Work out the finished part from the listing and answer in its coordinate system (mm). A direction names the side the tool comes from. Round coordinates to 2 decimals unless told otherwise and drop trailing zeros. Order: outer loops, then holes, each group sorted by start corner. A loop starts at its lowest first (then second) coordinate and runs counter-clockwise, first axis right, second up. Notation, with made-up numbers: M 80,-20 L 108,-20 A31 ccw 108,14 Z; hole C 89,86.25 d6. An arc over 180 degrees is marked long. Return JSON: item names as keys, results as strings.
from build123d import *

# Parameters (mm, degrees)
CYLINDER074_R          = 2
CYLINDER074_DEPTH      = 10
CYLINDER073_R          = 2
CYLINDER073_DEPTH      = 10
CYLINDER075_R          = 2
CYLINDER075_DEPTH      = 10
CYLINDER076_R          = 2
CYLINDER076_DEPTH      = 10
BOX103_W               = 1
BOX103_H               = 100
BOX103_DEPTH           = 5
BOX102_W               = 1
BOX102_H               = 100
BOX102_DEPTH           = 5
BOX100_W               = 2
BOX100_H               = 2
BOX100_DEPTH           = 80
BOX100_PLACEMENT_ANGLE = 45
BOX101_W               = 2
BOX101_H               = 2
BOX101_DEPTH           = 80
BOX101_PLACEMENT_ANGLE = 45
BOX097_W               = 2
BOX097_H               = 2
BOX097_DEPTH           = 80
BOX097_PLACEMENT_ANGLE = 45
BOX096_W               = 2
BOX096_H               = 2
BOX096_DEPTH           = 80
BOX096_PLACEMENT_ANGLE = 45
BOX095_W               = 2
BOX095_H               = 2
BOX095_DEPTH           = 80
BOX095_PLACEMENT_ANGLE = 45
BOX094_W               = 2
BOX094_H               = 2
BOX094_DEPTH           = 80
BOX094_PLACEMENT_ANGLE = 45
BOX093_W               = 2
BOX093_H               = 2
BOX093_DEPTH           = 80
BOX093_PLACEMENT_ANGLE = 45
BOX092_W               = 2
BOX092_H               = 2
BOX092_DEPTH           = 80
BOX092_PLACEMENT_ANGLE = 45
BOX091_W               = 2
BOX091_H               = 2
BOX091_DEPTH           = 80
BOX091_PLACEMENT_ANGLE = 45
BOX090_W               = 2
BOX090_H               = 2
BOX090_DEPTH           = 80
BOX090_PLACEMENT_ANGLE = 45
BOX089_W               = 2
BOX089_H               = 2
BOX089_DEPTH           = 80
BOX089_PLACEMENT_ANGLE = 45
BOX088_W               = 2
BOX088_H               = 2
BOX088_DEPTH           = 80
BOX088_PLACEMENT_ANGLE = 45
BOX087_W               = 2
BOX087_H               = 2
BOX087_DEPTH           = 80
BOX087_PLACEMENT_ANGLE = 45
BOX086_W               = 2
BOX086_H               = 2
BOX086_DEPTH           = 80
BOX086_PLACEMENT_ANGLE = 45
BOX084_W               = 2
BOX084_H               = 2
BOX084_DEPTH           = 80
BOX084_PLACEMENT_ANGLE = 45
BOX085_W               = 2
BOX085_H               = 2
BOX085_DEPTH           = 80
BOX085_PLACEMENT_ANGLE = 45
BOX099_W               = 2
BOX099_H               = 2
BOX099_DEPTH           = 80
BOX099_PLACEMENT_ANGLE = 45
BOX098_W               = 2
BOX098_H               = 50
BOX098_DEPTH           = 50
PAD014_DEPTH           = 5
BOX083_W               = 2
BOX083_H               = 93
BOX083_DEPTH           = 130
CUT076_PLACEMENT_ANGLE = 90


with BuildPart() as cylinder043:
    # Cylinder074 → Cylinder074 (new body)
    with BuildSketch(Plane(origin=(102, 0, 27), x_dir=(1, 0, 0), z_dir=(0, -1, 0))):
        Circle(CYLINDER074_R)
    extrude(amount=CYLINDER074_DEPTH)


with BuildPart() as cylinder042:
    # Cylinder073 → Cylinder073 (new body)
    with BuildSketch(Plane(origin=(19.8, 0, 27), x_dir=(1, 0, 0), z_dir=(0, -1, 0))):
        Circle(CYLINDER073_R)
    extrude(amount=CYLINDER073_DEPTH)


with BuildPart() as cylinder044:
    # Cylinder075 → Cylinder075 (new body)
    with BuildSketch(Plane(origin=(102, 0, 143), x_dir=(1, 0, 0), z_dir=(0, -1, 0))):
        Circle(CYLINDER075_R)
    extrude(amount=CYLINDER075_DEPTH)


with BuildPart() as obj1:
    # Cylinder076 → Cylinder076 (new body)
    with BuildSketch(Plane(origin=(32.2, 0, 143), x_dir=(1, 0, 0), z_dir=(0, -1, 0))):
        Circle(CYLINDER076_R)
    extrude(amount=CYLINDER076_DEPTH)

    # Fusion045: union Cylinder043, Cylinder042, Cylinder044
    add(cylinder043.part)
    add(cylinder042.part)
    add(cylinder044.part)


with BuildPart() as obj1_1:
    # Fusion045 placement: moved
    add(obj1.part.moved(Location((0, 5, 0))))


with BuildPart() as cube094:
    # Box103 → Box103 (new body)
    with BuildSketch(Plane.XY.offset(125)):
        with Locations((0.5, 50)):
            Rectangle(BOX103_W, BOX103_H)
    extrude(amount=BOX103_DEPTH)


with BuildPart() as obj2:
    # Box102 → Box102 (new body)
    with BuildSketch(Plane.XY):
        with Locations((0.5, 50)):
            Rectangle(BOX102_W, BOX102_H)
    extrude(amount=BOX102_DEPTH)

    # Fusion044: union Cube094
    add(cube094.part)


with BuildPart() as cube091:
    # Box100 → Box100 (new body)
    with BuildSketch(Plane.XY):
        with Locations((1, 1)):
            Rectangle(BOX100_W, BOX100_H)
    extrude(amount=BOX100_DEPTH)


with BuildPart() as cube091_1:
    # Box100 placement: moved
    add(cube091.part.moved(Location((0, 90, 0))).rotate(Axis((0, 90, 0), (-1, 0, 0)), BOX100_PLACEMENT_ANGLE))


with BuildPart() as cube092:
    # Box101 → Box101 (new body)
    with BuildSketch(Plane.XY):
        with Locations((1, 1)):
            Rectangle(BOX101_W, BOX101_H)
    extrude(amount=BOX101_DEPTH)


with BuildPart() as cube092_1:
    # Box101 placement: moved
    add(cube092.part.moved(Location((0, 96, 0))).rotate(Axis((0, 96, 0), (-1, 0, 0)), BOX101_PLACEMENT_ANGLE))


with BuildPart() as cube088:
    # Box097 → Box097 (new body)
    with BuildSketch(Plane.XY):
        with Locations((1, 1)):
            Rectangle(BOX097_W, BOX097_H)
    extrude(amount=BOX097_DEPTH)


with BuildPart() as cube088_1:
    # Box097 placement: moved
    add(cube088.part.moved(Location((0, 78, 0))).rotate(Axis((0, 78, 0), (-1, 0, 0)), BOX097_PLACEMENT_ANGLE))


with BuildPart() as cube087:
    # Box096 → Box096 (new body)
    with BuildSketch(Plane.XY):
        with Locations((1, 1)):
            Rectangle(BOX096_W, BOX096_H)
    extrude(amount=BOX096_DEPTH)


with BuildPart() as cube087_1:
    # Box096 placement: moved
    add(cube087.part.moved(Location((0, 72, 0))).rotate(Axis((0, 72, 0), (-1, 0, 0)), BOX096_PLACEMENT_ANGLE))


with BuildPart() as cube086:
    # Box095 → Box095 (new body)
    with BuildSketch(Plane.XY):
        with Locations((1, 1)):
            Rectangle(BOX095_W, BOX095_H)
    extrude(amount=BOX095_DEPTH)


with BuildPart() as cube086_1:
    # Box095 placement: moved
    add(cube086.part.moved(Location((0, 66, 0))).rotate(Axis((0, 66, 0), (-1, 0, 0)), BOX095_PLACEMENT_ANGLE))


with BuildPart() as cube085:
    # Box094 → Box094 (new body)
    with BuildSketch(Plane.XY):
        with Locations((1, 1)):
            Rectangle(BOX094_W, BOX094_H)
    extrude(amount=BOX094_DEPTH)


with BuildPart() as cube085_1:
    # Box094 placement: moved
    add(cube085.part.moved(Location((0, 60, 0))).rotate(Axis((0, 60, 0), (-1, 0, 0)), BOX094_PLACEMENT_ANGLE))


with BuildPart() as cube084:
    # Box093 → Box093 (new body)
    with BuildSketch(Plane.XY):
        with Locations((1, 1)):
            Rectangle(BOX093_W, BOX093_H)
    extrude(amount=BOX093_DEPTH)


with BuildPart() as cube084_1:
    # Box093 placement: moved
    add(cube084.part.moved(Location((0, 54, 0))).rotate(Axis((0, 54, 0), (-1, 0, 0)), BOX093_PLACEMENT_ANGLE))


with BuildPart() as cube083:
    # Box092 → Box092 (new body)
    with BuildSketch(Plane.XY):
        with Locations((1, 1)):
            Rectangle(BOX092_W, BOX092_H)
    extrude(amount=BOX092_DEPTH)


with BuildPart() as cube083_1:
    # Box092 placement: moved
    add(cube083.part.moved(Location((0, 48, 0))).rotate(Axis((0, 48, 0), (-1, 0, 0)), BOX092_PLACEMENT_ANGLE))


with BuildPart() as cube082:
    # Box091 → Box091 (new body)
    with BuildSketch(Plane.XY):
        with Locations((1, 1)):
            Rectangle(BOX091_W, BOX091_H)
    extrude(amount=BOX091_DEPTH)


with BuildPart() as cube082_1:
    # Box091 placement: moved
    add(cube082.part.moved(Location((0, 42, 0))).rotate(Axis((0, 42, 0), (-1, 0, 0)), BOX091_PLACEMENT_ANGLE))


with BuildPart() as cube081:
    # Box090 → Box090 (new body)
    with BuildSketch(Plane.XY):
        with Locations((1, 1)):
            Rectangle(BOX090_W, BOX090_H)
    extrude(amount=BOX090_DEPTH)


with BuildPart() as cube081_1:
    # Box090 placement: moved
    add(cube081.part.moved(Location((0, 36, 0))).rotate(Axis((0, 36, 0), (-1, 0, 0)), BOX090_PLACEMENT_ANGLE))


with BuildPart() as cube080:
    # Box089 → Box089 (new body)
    with BuildSketch(Plane.XY):
        with Locations((1, 1)):
            Rectangle(BOX089_W, BOX089_H)
    extrude(amount=BOX089_DEPTH)


with BuildPart() as cube080_1:
    # Box089 placement: moved
    add(cube080.part.moved(Location((0, 30, 0))).rotate(Axis((0, 30, 0), (-1, 0, 0)), BOX089_PLACEMENT_ANGLE))


with BuildPart() as cube079:
    # Box088 → Box088 (new body)
    with BuildSketch(Plane.XY):
        with Locations((1, 1)):
            Rectangle(BOX088_W, BOX088_H)
    extrude(amount=BOX088_DEPTH)


with BuildPart() as cube079_1:
    # Box088 placement: moved
    add(cube079.part.moved(Location((0, 24, 0))).rotate(Axis((0, 24, 0), (-1, 0, 0)), BOX088_PLACEMENT_ANGLE))


with BuildPart() as cube078:
    # Box087 → Box087 (new body)
    with BuildSketch(Plane.XY):
        with Locations((1, 1)):
            Rectangle(BOX087_W, BOX087_H)
    extrude(amount=BOX087_DEPTH)


with BuildPart() as cube078_1:
    # Box087 placement: moved
    add(cube078.part.moved(Location((0, 18, 0))).rotate(Axis((0, 18, 0), (-1, 0, 0)), BOX087_PLACEMENT_ANGLE))


with BuildPart() as cube077:
    # Box086 → Box086 (new body)
    with BuildSketch(Plane.XY):
        with Locations((1, 1)):
            Rectangle(BOX086_W, BOX086_H)
    extrude(amount=BOX086_DEPTH)


with BuildPart() as cube077_1:
    # Box086 placement: moved
    add(cube077.part.moved(Location((0, 12, 0))).rotate(Axis((0, 12, 0), (-1, 0, 0)), BOX086_PLACEMENT_ANGLE))


with BuildPart() as cube075:
    # Box084 → Box084 (new body)
    with BuildSketch(Plane.XY):
        with Locations((1, 1)):
            Rectangle(BOX084_W, BOX084_H)
    extrude(amount=BOX084_DEPTH)


with BuildPart() as cube075_1:
    # Box084 placement: moved
    add(cube075.part.rotate(Axis((0, 0, 0), (-1, 0, 0)), BOX084_PLACEMENT_ANGLE))


with BuildPart() as cube076:
    # Box085 → Box085 (new body)
    with BuildSketch(Plane.XY):
        with Locations((1, 1)):
            Rectangle(BOX085_W, BOX085_H)
    extrude(amount=BOX085_DEPTH)


with BuildPart() as cube076_1:
    # Box085 placement: moved
    add(cube076.part.moved(Location((0, 6, 0))).rotate(Axis((0, 6, 0), (-1, 0, 0)), BOX085_PLACEMENT_ANGLE))


with BuildPart() as fusion043:
    # Box099 → Box099 (new body)
    with BuildSketch(Plane.XY):
        with Locations((1, 1)):
            Rectangle(BOX099_W, BOX099_H)
    extrude(amount=BOX099_DEPTH)


with BuildPart() as fusion043_1:
    # Box099 placement: moved
    add(fusion043.part.moved(Location((0, 84, 0))).rotate(Axis((0, 84, 0), (-1, 0, 0)), BOX099_PLACEMENT_ANGLE))

    # Fusion043: union Cube091, Cube092, Cube088, Cube087, Cube086, Cube085, Cube084, Cube083, Cube082, Cube081, Cube080, Cube079, Cube078, Cube077, Cube075, Cube076
    add(cube091_1.part)
    add(cube092_1.part)
    add(cube088_1.part)
    add(cube087_1.part)
    add(cube086_1.part)
    add(cube085_1.part)
    add(cube084_1.part)
    add(cube083_1.part)
    add(cube082_1.part)
    add(cube081_1.part)
    add(cube080_1.part)
    add(cube079_1.part)
    add(cube078_1.part)
    add(cube077_1.part)
    add(cube075_1.part)
    add(cube076_1.part)


with BuildPart() as obj3:
    # Box098 → Box098 (new body)
    with BuildSketch(Plane(origin=(0, 46, 0), x_dir=(1, 0, 0), z_dir=(0, 0, 1))):
        with Locations((1, 25)):
            Rectangle(BOX098_W, BOX098_H)
    extrude(amount=BOX098_DEPTH)

    # Cut074: cut Fusion043
    add(fusion043_1.part, mode=Mode.SUBTRACT)


with BuildPart() as obj3_1:
    # Cut074 placement: moved
    add(obj3.part.moved(Location((0, -20, 38))))


with BuildPart() as pad014:
    # Sketch021 → Pad014 (new body)
    with BuildSketch(Plane.YZ):
        Polygon((0, 0), (13.661518, 129.980665), (0, 129.980665), align=None)
    extrude(amount=PAD014_DEPTH)


with BuildPart() as obj4:
    # Box083 → Box083 (new body)
    with BuildSketch(Plane.XY):
        with Locations((1, 46.5)):
            Rectangle(BOX083_W, BOX083_H)
    extrude(amount=BOX083_DEPTH)

    # Cut073: cut Pad014
    add(pad014.part, mode=Mode.SUBTRACT)

    # Cut075: cut obj3
    add(obj3_1.part, mode=Mode.SUBTRACT)

    # Cut076: cut obj2
    add(obj2.part, mode=Mode.SUBTRACT)


with BuildPart() as obj4_1:
    # Cut076 placement: moved
    add(obj4.part.moved(Location((14.6, 2, 20))).rotate(Axis((14.6, 2, 20), (0, 0, -1)), CUT076_PLACEMENT_ANGLE))

    # Cut077: cut obj1
    add(obj1_1.part, mode=Mode.SUBTRACT)


with BuildPart() as part_mirroring011:
    # Part__Mirroring011: instance of obj4
    add(obj4_1.part.mirror(Plane(origin=(0, 0, 0), x_dir=(1, 0, 0), z_dir=(0, 1, 0))))


with BuildPart() as part_mirroring011_1:
    # Part__Mirroring011 placement: moved
    add(part_mirroring011.part.moved(Location((0, 110, 0))))


solid = part_mirroring011_1.part
Item 1: Consider line 1 along X through (y, z) = (109.45, 27); line 2 along X through (y, z) = (109.6, 143); line 3 along X through (y, z) = (109.1, 34.5). Determine where each line is inside the solid, lowest interval first. Write a range as [from, to].
Output:
{"line 1": "x = [15.34, 17.8], [21.8, 100], [104, 107.6]", "line 2": "x = [27.53, 30.2], [34.2, 100], [104, 107.6]", "line 3": "x = [16.12, 107.6]"}
Item 2: The mould has two halves that part along X. Classify faces 1 (the flat face through (84.5, 109, 63.9)), 2 (the flat face through (71, 108, 84)): pulls with the +X half, pulls with the -X half, needs draft (parallel to the pull), parting line crosses it, or undercut.
Output:
{"face 1": "undercut", "face 2": "needs draft"}
Item 3: Find section D-D (z = 143). Determine the outline of the cut face in (x, y), plus the area to 3 significant figures.
Output:
{"outline": "M 27.53,108 L 30.2,108 L 30.2,110 L 27.53,110 Z; M 34.2,108 L 100,108 L 100,110 L 34.2,110 Z; M 104,108 L 107.6,108 L 107.6,110 L 104,110 Z", "area": "144 mm^2"}
Item 4: Which of the six approach directions +Z, -Z, +X, -X, +Y, -Y give full straight-line access (tool end or side, diameter ignored) to faces 3 (the flat face through (60, 109, 22)), 4 (the flat face through (55.8, 108.99, 92.37))?
Output:
{"face 3": "-Z, +X, -X, -Y", "face 4": "+Y, -Y"}
Item 5: Find section A-A (z = 27). Determine the outline of the cut face in (x, y).
Output:
{"outline": "M 15.34,108 L 17.8,108 L 17.8,110 L 15.34,110 Z; M 21.8,108 L 100,108 L 100,110 L 21.8,110 Z; M 104,108 L 107.6,108 L 107.6,110 L 104,110 Z"}
Item 6: Each of these flat-tipped pins is pushed along its axis until it touches: pin 1 (1.1 mm diameter, centred on x = 104.5, y = 108.5, fed in from +Z); pin 2 (0.5 mm diameter, centred on x = 29.5, y = 108.5, fed in from +Z). Where does it stop, or does it pass through?
Output:
{"pin 1": "stops at z = 150", "pin 2": "stops at z = 145"}
Item 7: Find section B-B (x = 36). Determine the outline of the cut face in (y, z), plus the area to 3 significant figures.
Output:
{"outline": "M 108,25 L 109,25 L 109,20 L 110,20 L 110,150 L 109,150 L 109,145 L 108,145 Z", "area": "250 mm^2"}
